The figure shows three views and two pictorial views of one solid part (mm, origin at its lowest corner). Answer the questions. Coordinates: 2 decimals unless noted, no trailing zeros. Order: outer loops, then holes, each group sorted by start corner. A loop starts at its lowest first (then second) coordinate and runs counter-clockwise, first axis right, second up. Notation, with made-up numbers: (-34, 29.25) - (-14, 29.25) arc R25 cw to (-14, 57.25) - close; hole circle Ø9 at (-7, 35). An arc over 180 degrees is marked (long way). Use one line per item in the form item = value.
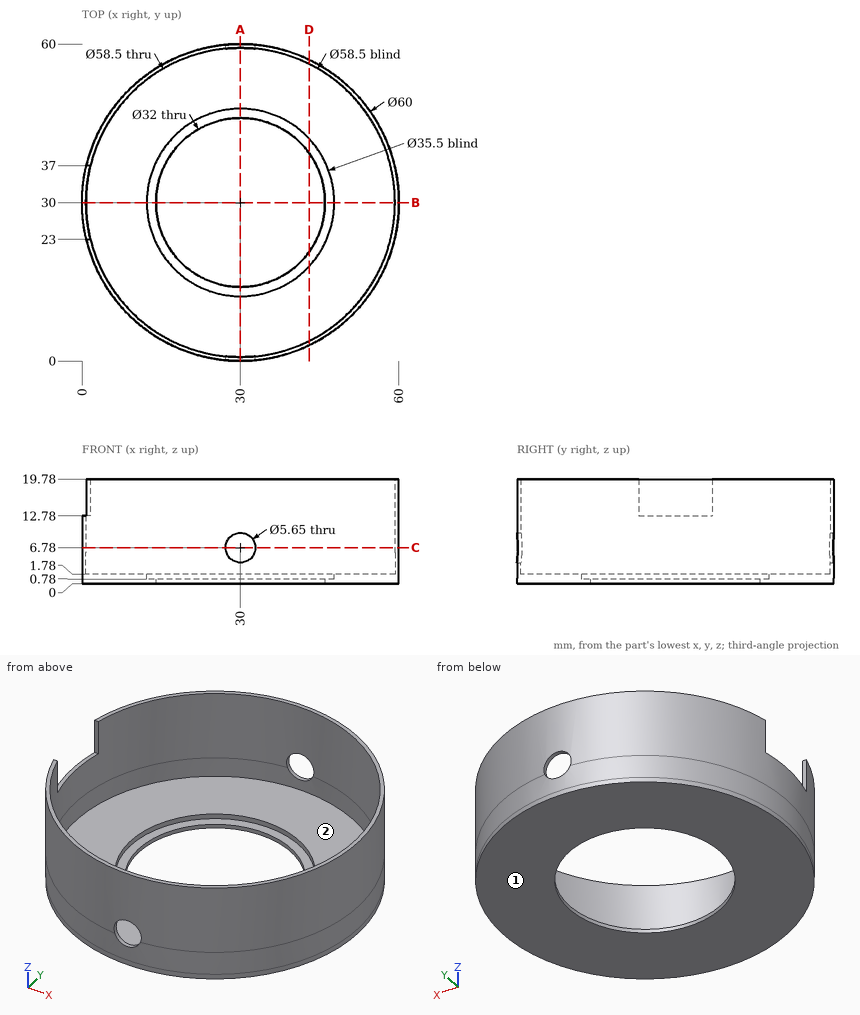
(1) Section C-C, the plane z = 6.78 is taken. Write down the section's boundary in (x, y) (3 decimals), then the cut area to 3 significant figures.
Answer list:
outline = (27.175, 0.133) - (27.175, 0.887) arc R29.25 cw to (27.175, 59.113) - (27.175, 59.867) arc R30 ccw to start; (32.825, 0.133) arc R30 ccw to (32.825, 59.867) - (32.825, 59.113) arc R29.25 cw to (32.825, 0.887) - close
area = 131 mm2
(2) Straight lines are drawn through the part: L1, parallel to Z at x = 30, y = 0.45 (3 decimals); L2, parallel to Y at x = 30, z = 13; L3, parallel to Y at x = 30, z = 1.45. For each, find the intervals that lie inside material, in ascending order.
Answer list:
L1 = 0 to 3.955, 9.605 to 19.78
L2 = 0 to 0.75, 59.25 to 60
L3 = 0 to 12.25, 47.75 to 60
(3) Section B-B, the plane y = 30 is taken. Write down the section's boundary in (x, z).
Answer list:
outline = (0, 0) - (14, 0) - (14, 0.78) - (12.25, 0.78) - (12.25, 1.78) - (0.75, 1.78) - (0.75, 12.78) - (0, 12.78) - close; (46, 0) - (60, 0) - (60, 19.78) - (59.25, 19.78) - (59.25, 1.78) - (47.75, 1.78) - (47.75, 0.78) - (46, 0.78) - close
(4) Section A-A, the plane x = 30 is taken. Write down the section's boundary in (y, z) (3 decimals), then the cut area to 3 significant figures.
Answer list:
outline = (0, 0) - (14, 0) - (14, 0.78) - (12.25, 0.78) - (12.25, 1.78) - (0.75, 1.78) - (0.75, 3.955) - (0, 3.955) - close; (0, 9.605) - (0.75, 9.605) - (0.75, 19.78) - (0, 19.78) - close; (46, 0) - (60, 0) - (60, 3.955) - (59.25, 3.955) - (59.25, 1.78) - (47.75, 1.78) - (47.75, 0.78) - (46, 0.78) - close; (59.25, 9.605) - (60, 9.605) - (60, 19.78) - (59.25, 19.78) - close
area = 64.9 mm2
(5) Given pin 1 Ø1.3 at (x, y) = (1, 31.5) entering from +Z; pin 2 Ø1 at (x, y) = (42, 11) entering from +Z; pin 3 Ø1.5 at (y, z) = (21.5, 12) entering from -X; pin 4 Ø18 at (x, y) = (35.5, 26) entering from +Z, each flat-ended and moving along its own axis, determine where each tip first touches the part or whether it passes through.
Answer list:
pin_1 = 12.78
pin_2 = 1.78
pin_3 = 1.02
pin_4 = through
(6) Section D-D, the plane x = 43 is taken. Write down the section's boundary in (y, z).
Answer list:
outline = (2.96, 0) - (20.67, 0) - (20.67, 0.78) - (17.91, 0.78) - (17.91, 1.78) - (3.8, 1.78) - (3.8, 19.78) - (2.96, 19.78) - close; (39.33, 0) - (57.04, 0) - (57.04, 19.78) - (56.2, 19.78) - (56.2, 1.78) - (42.09, 1.78) - (42.09, 0.78) - (39.33, 0.78) - close
(7) The mould has two halves that part along Y. Classify the marked faces 1 and 2: +Y half, -Y half, draft (parallel to the pull), parting line (faces both ways), or undercut.
Answer list:
face_1 = draft
face_2 = undercut
